CAD build for the part. Positions are in the model's coordinates, mm. Coordinates: 2 decimals unless noted, no trailing zeros. Loops run counter-clockwise (first coordinate to the right, second up) from the corner with the lowest first, then second, coordinate; pieces in that order, holes last. Notation, with made-up numbers: (-36.75, 19.25) -> (-23.75, 19.25) arc R17 ccw to (-23.75, 23.25) -> close; hole circle Ø11 at (27, 42.5). An arc over 180 degrees is marked (long way). Answer as CSV lines item,"result". Start each with the question number.
```python
from build123d import *

# Parameters (mm, degrees)
SKETCH1_W            = 56
SKETCH1_H            = 24
BOSS_EXTRUDE1_DEPTH  = 1.6
FILLET1_R            = 5
SKETCH2_R            = 2.1
CUT_EXTRUDE1_DEPTH   = 2.6
LPATTERN1_COUNT      = 7
LPATTERN1_PITCH      = 8
LPATTERN1_COUNT_DIR2 = 3
LPATTERN1_PITCH_DIR2 = 8


with BuildPart() as part:
    # Sketch1 → Boss-Extrude1 (new body)
    with BuildSketch(Plane(origin=(0, 0, 0), x_dir=(1, 0, 0), z_dir=(0, 1, 0))):
        with Locations((28, -12)):
            Rectangle(SKETCH1_W, SKETCH1_H)
    extrude(amount=BOSS_EXTRUDE1_DEPTH)

    # Fillet1
    fillet1_edges = [part.edges().sort_by_distance(p)[0] for p in [
        (0, 0.8, 0),
        (56, 0.8, 0),
        (56, 0.8, 24),
        (0, 0.8, 24),
    ]]
    fillet(fillet1_edges, radius=FILLET1_R)

    # Sketch2 → Cut-Extrude1 (cut, through all)
    with BuildSketch(Plane(origin=(0, 1.6, 0), x_dir=(1, 0, 0), z_dir=(0, 1, 0))):
        with Locations((4, -4)):
            Circle(SKETCH2_R)
    cut_extrude1 = extrude(amount=-CUT_EXTRUDE1_DEPTH, mode=Mode.SUBTRACT)

    # LPattern1: Cut-Extrude1 7 × 3
    with Locations(*[(i * LPATTERN1_PITCH, 0, j * LPATTERN1_PITCH_DIR2) for i in range(LPATTERN1_COUNT) for j in range(LPATTERN1_COUNT_DIR2) if (i, j) != (0, 0)]):
        add(cut_extrude1, mode=Mode.SUBTRACT)


solid = part.part
```
Q1. Two-plate mould, pull along Z, no slides. Class faces 1 (the cylindrical face through (43.727, 0.811, 17.918)), 2 (the flat face through (28, 1.6, 9)), 3 (the cylindrical face through (55, 1, 2)), 4 (the flat face through (28, 1, 24)): pulls with the +Z half, pulls with the -Z half, needs draft (parallel to the pull), parting line crosses it, or undercut.
Q2. Saw through at B-B (z = 12). Give the number of separate pieces and of enclosed holes in the cut face, and give its area (3 significant figures).
Q3. Probe probe 1 along Z at (x, y) = (12, 0.7); probe 2 along Z at (x, y) = (19.5, 1.55). List the from-to ranges inside material, lowest first. Write a range as from..to.
Q4. Saw through at A-A (x = 36). List the corners of the cut face in (y, z).
Q5. Saw through at D-D (x = 4). List the corners of the cut face in (y, z).
Q6. Pin check, flat tip, straight feed: pin 1 Ø3.5 at (x, z) = (52, 4) entering from +Y. Stop position of the tip, or through.
Ans:
1,face 1,"undercut"
1,face 2,"needs draft"
1,face 3,"pulls with the -Z half"
1,face 4,"pulls with the +Z half"
2,separate pieces,"8"
2,enclosed holes,"0"
2,area,"42.6 mm²"
3,probe 1,"z = 0..1.9, 6.1..9.9, 14.1..17.9, 22.1..24"
3,probe 2,"z = 0..1.96, 6.04..9.96, 14.04..17.96, 22.04..24"
4,outline,"(0, 0) -> (1.6, 0) -> (1.6, 1.9) -> (0, 1.9) -> close; (0, 6.1) -> (1.6, 6.1) -> (1.6, 9.9) -> (0, 9.9) -> close; (0, 14.1) -> (1.6, 14.1) -> (1.6, 17.9) -> (0, 17.9) -> close; (0, 22.1) -> (1.6, 22.1) -> (1.6, 24) -> (0, 24) -> close"
5,outline,"(0, 0.1) -> (1.6, 0.1) -> (1.6, 1.9) -> (0, 1.9) -> close; (0, 6.1) -> (1.6, 6.1) -> (1.6, 9.9) -> (0, 9.9) -> close; (0, 14.1) -> (1.6, 14.1) -> (1.6, 17.9) -> (0, 17.9) -> close; (0, 22.1) -> (1.6, 22.1) -> (1.6, 23.9) -> (0, 23.9) -> close"
6,pin 1,"passes through"
